Geometry: final body of the model. Coordinates: model frame, mm. Face numbers are marked on the shaded views. Coordinates: 2 decimals unless noted, no trailing zeros. Write each loop counter-clockwise with the first axis right and the second up, starting at its lowest first coordinate (ties: lowest second). Pieces come first, ordered by that corner, then holes. Notation, with made-up numbers: (-23, 44) -> (-16, 44) arc R16 cw to (-16, 55) -> close; hole circle Ø4 at (44.25, 88). An arc over 180 degrees is marked (long way). One line per item, written item: value. Start each with the question number.
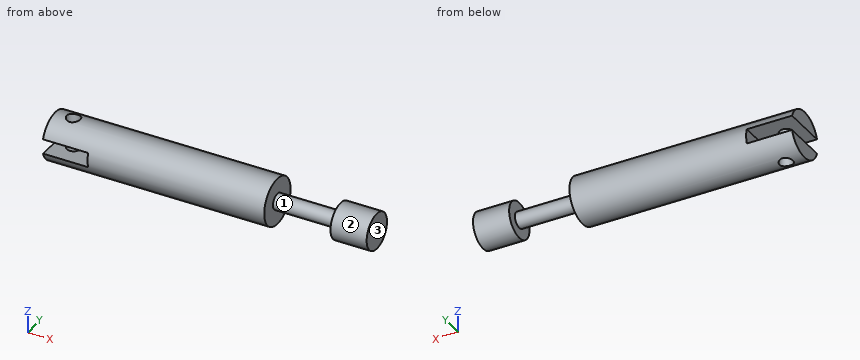
from build123d import *

# Parameters (mm, degrees)
SKETCH1_W          = 14
SKETCH1_H          = 1.75
CUT_EXTRUDE1_REACH = 12.35
SKETCH2_R          = 1.5
SKETCH3_W          = 3.25
SKETCH3_H          = 10.35
CUT_EXTRUDE2_DEPTH = 10


with BuildPart() as part:
    # Sketch1 → Revolve1 (revolve)
    with BuildSketch(Plane.XY):
        Polygon((0, 5.175), (0, 0), (49.1, 0), (49.1, 1.75), (49.1, 5.175), align=None)
        with Locations((56.1, 0.875)):
            Rectangle(SKETCH1_W, SKETCH1_H)
        Polygon((63.1, 1.75), (63.1, 0), (71.1, 0), (71.1, 4), (63.1, 4), align=None)
    revolve(axis=Axis((0, 0, 0), (1, 0, 0)))

    # Sketch2 → Cut-Extrude1 (cut, up to next)
    with BuildSketch(Plane.XY.offset(5.175), mode=Mode.PRIVATE) as cut_extrude1_sk1:
        with Locations((4, 0)):
            Circle(SKETCH2_R)
    cut_extrude1_tool1 = extrude(cut_extrude1_sk1.sketch, amount=-CUT_EXTRUDE1_REACH, mode=Mode.PRIVATE) & part.part
    add(cut_extrude1_tool1.solids().sort_by_distance((4, 0, 5.175))[0], mode=Mode.SUBTRACT)

    # Sketch3 → Cut-Extrude2 (cut)
    with BuildSketch(Plane.ZY):
        Rectangle(SKETCH3_W, SKETCH3_H)
    extrude(amount=-CUT_EXTRUDE2_DEPTH, mode=Mode.SUBTRACT)


solid = part.part
Q1. Cut plane A-A on y = 0. Output: boundary loops of the cut face in (x, z) (3 decimals).
Q2. Draft query along X for the marked faces 1, 2 and 3. Return one class per face: pulls with the +X half, pulls with the -X half, needs draft (parallel to the pull), parting line crosses it, or undercut.
Q3. Cut plane C-C on x = 4. Output: boundary loops of the cut face in (y, z) (3 decimals), and give its area (3 significant figures).
Q4. Cut plane B-B on z = 0. Output: boundary loops of the cut face in (x, y) (3 decimals), and give its area (3 significant figures).
Q5. First-contact query: P1, Ø1.5, axis at x = 8.5, z = 2.5, coming from the +Y side. Flat tip, straight axial feed; report the tip coordinate or a pass-through.
Q6. Cut plane D-D on x = 61.5. Output: boundary loops of the cut face in (y, z).
Q7. Line query: L1, parallel to X at y = 0, z = -4.35; L2, parallel to X at y = 0, z = 3.4; L3, parallel to X at y = -2, z = 1.5. Output: solid intervals per line, ascending. Write a range as from..to.
Solution:
1. outline: (0, -5.175) -> (2.5, -5.175) -> (2.5, -1.625) -> (0, -1.625) -> close; (0, 1.625) -> (2.5, 1.625) -> (2.5, 5.175) -> (0, 5.175) -> close; (5.5, -5.175) -> (49.1, -5.175) -> (49.1, -1.75) -> (63.1, -1.75) -> (63.1, -4) -> (71.1, -4) -> (71.1, 4) -> (63.1, 4) -> (63.1, 1.75) -> (49.1, 1.75) -> (49.1, 5.175) -> (5.5, 5.175) -> (5.5, 1.625) -> (10, 1.625) -> (10, -1.625) -> (5.5, -1.625) -> close
2. face 1: undercut
2. face 2: needs draft
2. face 3: pulls with the +X half
3. outline: (-4.913, -1.625) arc R5.175 ccw to (-1.5, -4.953) -> (-1.5, -1.625) -> close; (-4.913, 1.625) -> (-1.5, 1.625) -> (-1.5, 4.953) arc R5.175 ccw to start; (1.5, -4.953) arc R5.175 ccw to (4.913, -1.625) -> (1.5, -1.625) -> close; (1.5, 1.625) -> (4.913, 1.625) arc R5.175 ccw to (1.5, 4.953) -> close
3. area: 30.2 mm²
4. outline: (10, -5.175) -> (49.1, -5.175) -> (49.1, -1.75) -> (63.1, -1.75) -> (63.1, -4) -> (71.1, -4) -> (71.1, 4) -> (63.1, 4) -> (63.1, 1.75) -> (49.1, 1.75) -> (49.1, 5.175) -> (10, 5.175) -> close
4. area: 518 mm²
5. P1: y = 4.87
6. outline: circle Ø3.5 at (0, 0)
7. L1: 0..2.5, 5.5..49.1
7. L2: 0..2.5, 5.5..49.1, 63.1..71.1
7. L3: 10..49.1, 63.1..71.1
